from build123d import *

# Parameters (mm, degrees)
F2_ANGLE_BACK = 60
F2_ANGLE      = 120
F3_W          = 160
F3_H          = 4.7
F4_DEPTH      = 3
F5_T          = -2.5
F7_DEPTH      = 5
F8_W          = 5
F8_H          = 3
F9_DEPTH      = 99.0080415552
F10_W         = 16
F10_H         = 2.5
F11_DEPTH     = 25


with BuildPart() as f2:
    # F0 (on Front) → F2 (revolve)
    with BuildSketch(Plane.XZ, mode=Mode.PRIVATE) as f2_sk:
        Polygon((38, 20), (38, 0), (85, 0), (120, 16), (120, 20), align=None)
    revolve(f2_sk.sketch.rotate(Axis((0, 0, 35.0643768907), (0, 0, 1)), -F2_ANGLE_BACK), axis=Axis((0, 0, 35.0643768907), (0, 0, 1)), revolution_arc=F2_ANGLE)

    # F3 (on Top) → F4 (cut)
    with BuildSketch(Plane.XY):
        with Locations((80, 0)):
            Rectangle(F3_W, F3_H)
    extrude(amount=F4_DEPTH, mode=Mode.SUBTRACT)

    # F5
    f5_openings = [f2.faces().sort_by_distance(p)[0] for p in [
        (71.198195, 0, 20),
    ]]
    offset(amount=F5_T, openings=f5_openings, kind=Kind.INTERSECTION)

    # F6 (on face) → F7 (join)
    with BuildSketch(Plane.XY.offset(2.5)):
        with BuildLine():
            ThreePointArc((30.3829536253, -26.7792107614), (35.0740288533, -20.25), (38.3829536253, -12.9228043008))
            Line((38.3829536253, -12.9228043008), (37.3419780457, -12.3217967697))
            Line((37.3419780457, -12.3217967697), (29.3419780457, -26.1782032303))
            Line((29.3419780457, -26.1782032303), (30.3829536253, -26.7792107614))
        make_face()
        with BuildLine():
            Line((58.9926131403, -24.8217967697), (38.3829536253, -12.9228043008))
            ThreePointArc((38.3829536253, -12.9228043008), (35.0740288533, -20.25), (30.3829536253, -26.7792107614))
            Line((30.3829536253, -26.7792107614), (50.9926131403, -38.6782032303))
            Line((50.9926131403, -38.6782032303), (58.9926131403, -24.8217967697))
        make_face()
    extrude(amount=F7_DEPTH)

    # F8 (on face) → F9 (cut, through all)
    with BuildSketch(Plane(origin=(54.9926131403, -31.75, 0), x_dir=(0.5, 0.8660254038, 0), z_dir=(0.8660254038, -0.5, 0))):
        with Locations((0, 9)):
            Rectangle(F8_W, F8_H)
    extrude(amount=-F9_DEPTH, mode=Mode.SUBTRACT)

    # F10 (on face) → F11 (cut)
    with BuildSketch(Plane(origin=(54.9926131403, -31.75, 0), x_dir=(0.5, 0.8660254038, 0), z_dir=(0.8660254038, -0.5, 0))):
        with Locations((0, 8.75)):
            Rectangle(F10_W, F10_H)
    extrude(amount=-F11_DEPTH, mode=Mode.SUBTRACT)


solid = f2.part
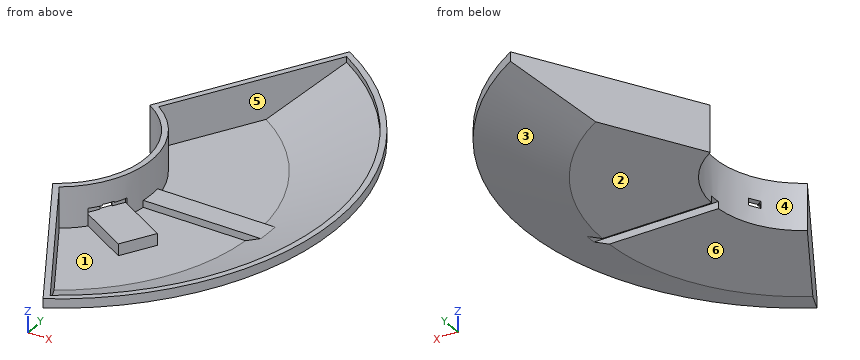
CAD build for the part. Positions are in the model's coordinates, mm. Face numbers are marked on the shaded views. A direction names the side the tool comes from. Round coordinates to 2 decimals unless told otherwise and drop trailing zeros. Write each loop counter-clockwise with the first axis right and the second up, starting at its lowest first coordinate (ties: lowest second). Pieces come first, ordered by that corner, then holes.
(1) Slice it at A-A, the plane z = 12.5. Write the cut outline in (x, y).
(2) 3-axis set-ups, long thin cutter, end or side, ignore diameter. For the marked faces 1 and 2: which of +Z, -Z, +X, -X, +Y, -Y reach the whole face in a straight line?
(3) Drop flat-ended pins along their axis: P1, Ø5, axis at x = 66.5, y = 1.5, coming from the +Z side; P2, Ø8, axis at x = 33, z = 4.5, coming from the +Y side; P3, Ø3, axis at y = -4.5, z = 3, coming from the -X side. Give the stop position or say it passes through.
(4) Probe line 1 along Z through (x, y) = (57, 44); line 2 along X through (y, z) = (49, 14.75); line 3 along X through (y, z) = (60, 18.5). List the from-to ranges inside material, lowest first.
(5) Mould opens along X. For the marked faces 3, 4, 5 and 6 say: pulls with the +X half, pulls with the -X half, needs draft (parallel to the pull), parting line crosses it, or undercut.
From the geometry:
1. outline: (19, -32.91) - (56.17, -97.29) arc R112.34 ccw to (56.17, 97.29) - (19, 32.91) arc R38 cw to start; hole (22.38, -33.76) - (55.32, -90.81) arc R106.33 ccw to (55.32, 90.81) - (22.38, 33.76) arc R40.5 cw to start
2. face 1: +Z
2. face 2: -Z, +X, -X, +Y, -Y
3. P1: stops at z = 5.5
3. P2: stops at y = 64.09
3. P3: stops at x = 37.52
4. line 1: z = 0 to 2.5
4. line 2: x = 28.29 to 31.18, 99.88 to 106.54
4. line 3: x = 34.64 to 37.53, 101.03 to 103.92
5. face 3: pulls with the +X half
5. face 4: pulls with the -X half
5. face 5: undercut
5. face 6: needs draft
